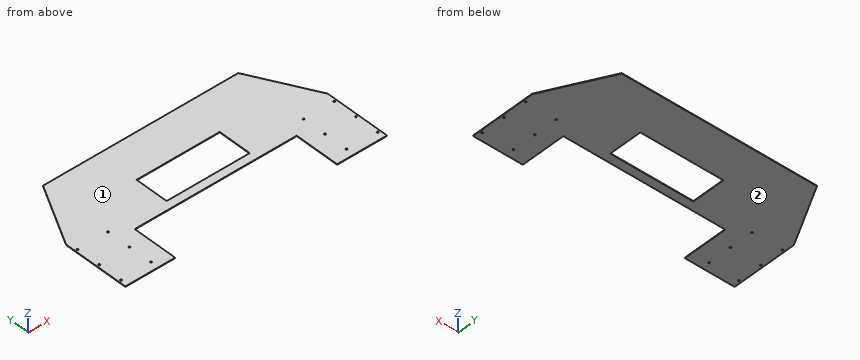
```python
from build123d import *

# Parameters (mm, degrees)
BASE_FLANGE1_DEPTH = 1.6002
SKETCH2_R          = 2.413
CUT_EXTRUDE1_DEPTH = 781.091023438
SKETCH3_W          = 254
SKETCH3_H          = 101.6
CUT_EXTRUDE2_DEPTH = 781.091023438


# Sheet-metal steps are written as plain solids
with BuildPart() as part:
    # Sketch1 → Base-Flange1 (new body)
    with BuildSketch(Plane.XY):
        Polygon((-76.2, -100.203), (76.2, -100.203), (76.2, 36.703), (571.5, 36.703), (571.5, -100.203), (723.9, -100.203), (723.9, 100.203), (622.3, 290.703), (25.4, 290.703), (-76.2, 100.203), align=None)
    extrude(amount=-BASE_FLANGE1_DEPTH)

    # Sketch2 → Cut-Extrude1 (cut, through all)
    with BuildSketch(Plane.XY):
        with Locations((24.637999896, 69.8754)):
            Circle(SKETCH2_R)
        with Locations((-68.6816, 69.8754)):
            Circle(SKETCH2_R)
        with Locations((24.637999896, -2.4638)):
            Circle(SKETCH2_R)
        with Locations((-68.6816, -3.6322)):
            Circle(SKETCH2_R)
        with Locations((-68.6816, -77.1398)):
            Circle(SKETCH2_R)
        with Locations((24.637999896, -74.803)):
            Circle(SKETCH2_R)
    cut_extrude1 = extrude(amount=-CUT_EXTRUDE1_DEPTH, mode=Mode.SUBTRACT)

    # Mirror1: Cut-Extrude1 across plane
    add(cut_extrude1.mirror(Plane.ZY.offset(-323.85)), mode=Mode.SUBTRACT)

    # Sketch3 → Cut-Extrude2 (cut, through all)
    with BuildSketch(Plane(origin=(0, 0, -1.6002), x_dir=(-1, 0, 0), z_dir=(0, 0, -1))):
        with Locations((-323.85, 112.903)):
            Rectangle(SKETCH3_W, SKETCH3_H)
    extrude(amount=-CUT_EXTRUDE2_DEPTH, mode=Mode.SUBTRACT)


solid = part.part
```
Check sheet for the modelled part. Datum: model origin and axes. Units: mm. Face numbers are marked on the shaded views. Give positions to 0.01 mm unless a question says otherwise; leave off trailing zeros. Loops run counter-clockwise (first coordinate to the right, second up) from the corner with the lowest first, then second, coordinate; pieces in that order, holes last. Notation, with made-up numbers: M -5.5,-15.5 L 14.5,-15.5 A15 ccw 14.5,12.5 Z; hole C 54,19.5 d9. An arc over 180 degrees is marked long. Answer in a Markdown table with one row per item.
1) Mould release check, pull along Z, two halves, no side actions. Record for the marked faces 1 and 2: released by +Z, released by -Z, zero draft, split by the parting line, or undercut.
Solutions:
| item | result |
|---|---|
| face 1 | released by +Z |
| face 2 | released by -Z |
2) Depth check by flat-ended pin: pin 1 (4 mm diameter, centred on x = 623.06, y = -2.46, fed in from -Z); pin 2 (0.8 mm diameter, centred on y = 131, z = -0.5, fed in from +X); pin 3 (0.8 mm diameter, centred on y = 128.5, z = -1, fed in from -X). Enter the tip coordinate at first touch or a pass-through.
Solutions:
| item | result |
|---|---|
| pin 1 | passes through |
| pin 2 | stops at x = 707.69 |
| pin 3 | stops at x = -61.32 |
3) Cross-section at C-C (z = -1). Count the separate pieces of the cut face and the enclosed holes in it, plus the area to 3 significant figures.
Solutions:
| item | result |
|---|---|
| separate pieces | 1 |
| enclosed holes | 13 |
| area | 200,000 mm^2 |
4) Thickness scan on line 1 (Y direction, x = 286.5, z = -0.3); line 2 (X direction, y = -37, z = -0.65); line 3 (X direction, y = 93, z = -1.35). Record the ranges inside material, lowest first.
Solutions:
| item | result |
|---|---|
| line 1 | y = 36.7 to 62.1, 163.7 to 290.7 |
| line 2 | x = -76.2 to 76.2, 571.5 to 723.9 |
| line 3 | x = -76.2 to 196.85, 450.85 to 723.9 |
5) Cross-section at B-B (y = -18). Enter the section's corners in (x, z).
Solutions:
| item | result |
|---|---|
| outline | M -76.2,-1.6 L 76.2,-1.6 L 76.2,0 L -76.2,0 Z; M 571.5,-1.6 L 723.9,-1.6 L 723.9,0 L 571.5,0 Z |
6) Cross-section at A-A (x = 313). Enter the section's corners in (y, z).
Solutions:
| item | result |
|---|---|
| outline | M 36.7,-1.6 L 62.1,-1.6 L 62.1,0 L 36.7,0 Z; M 163.7,-1.6 L 290.7,-1.6 L 290.7,0 L 163.7,0 Z |
7) Cross-section at D-D (x = 504.5). Enter the section's corners in (y, z), plus the area to 3 significant figures.
Solutions:
| item | result |
|---|---|
| outline | M 36.7,-1.6 L 290.7,-1.6 L 290.7,0 L 36.7,0 Z |
| area | 406 mm^2 |
